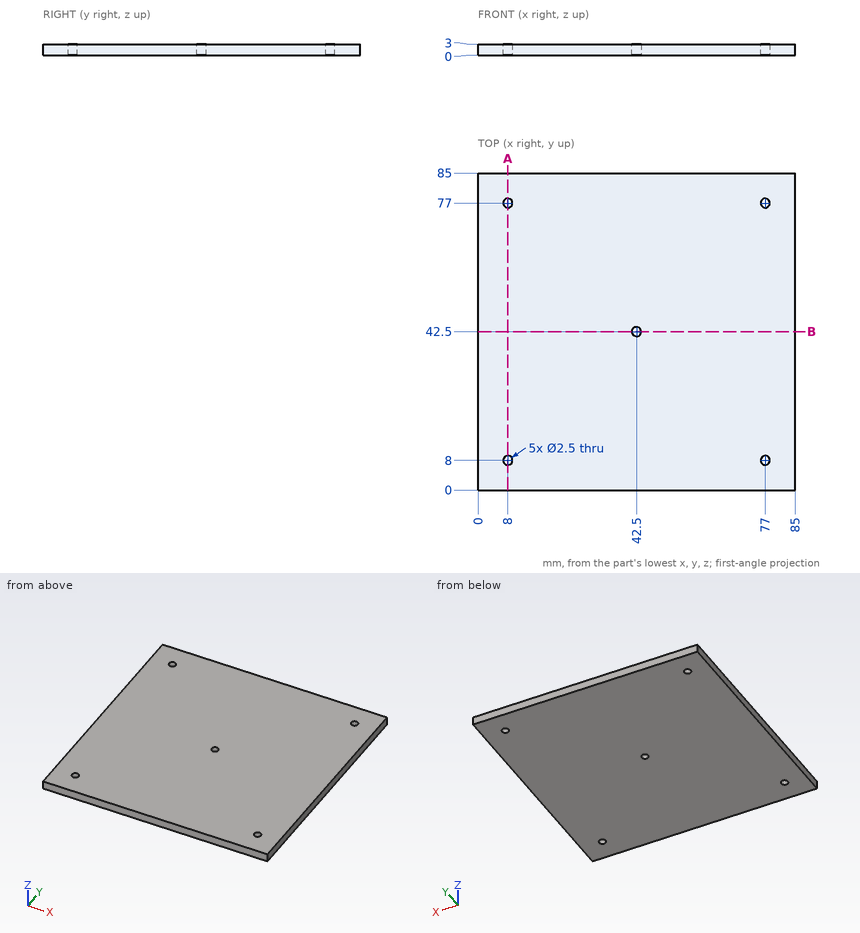
Input: dimensioned drawing with shaded views. Units: mm. Origin: part minimum x, y, z. Coordinates: 2 decimals unless noted, no trailing zeros. Order: outer loops, then holes, each group sorted by start corner. A loop starts at its lowest first (then second) coordinate and runs counter-clockwise, first axis right, second up.
Item 1: Section query A-A (x = 8). Output: boundary loops of the cut face in (y, z).
Answer:
outline: (0, 0) - (6.75, 0) - (6.75, 3) - (0, 3) - close; (9.25, 0) - (75.75, 0) - (75.75, 3) - (9.25, 3) - close; (78.25, 0) - (85, 0) - (85, 3) - (78.25, 3) - close
Item 2: Section query B-B (y = 42.5). Output: boundary loops of the cut face in (x, z), then the cut area to 4 significant figures.
Answer:
outline: (0, 0) - (41.25, 0) - (41.25, 3) - (0, 3) - close; (43.75, 0) - (85, 0) - (85, 3) - (43.75, 3) - close
area: 247.5 mm2
Item 3: Material intervals for line 1 along X through (y, z) = (77, 2.05); line 2 along Y through (x, z) = (42.5, 1.45), sorted ascending.
Answer:
line 1: x = 0 to 6.75, 9.25 to 75.75, 78.25 to 85
line 2: y = 0 to 41.25, 43.75 to 85
Item 4: Contact query for a flat-ended pin moving along its axis: P1, Ø4, axis at x = 42.5, y = 42.5, coming from the -Z side. Output: stop coordinate, or through.
Answer:
P1: stops at z = 0
